```python
from build123d import *

# Parameters (mm, degrees)
F1_DEPTH = 25
F4_D     = 5.5
F3_R     = 11
F5_DEPTH = 4


with BuildPart() as f1:
    # F0 (on Front) → F1 (new body, symmetric)
    with BuildSketch(Plane.XZ):
        with BuildLine():
            Line((23.3431457505, 0), (0, 0))
            Line((0, 0), (0, -4))
            Line((0, -4), (25, -4))
            ThreePointArc((25, -4), (26.5307337295, -3.69551813), (27.8284271247, -2.8284271247))
            Line((27.8284271247, -2.8284271247), (148.0365799265, 117.379725677))
            Line((148.0365799265, 117.379725677), (145.2081528017, 120.2081528017))
            Line((145.2081528017, 120.2081528017), (26.1715728753, 1.1715728753))
            ThreePointArc((26.1715728753, 1.1715728753), (24.87387948, 0.30448187), (23.3431457505, 0))
        make_face()
    extrude(amount=F1_DEPTH, both=True)

    # F2: F1 across plane


with BuildPart() as f1_1:
    add(f1.part)
    add(f1.part.mirror(Plane.YZ))

    # F4 (through all)
    with Locations(Plane.XY):
        with Locations((-17.45, 0), (8.725, -15.112143296), (8.725, 15.112143296)):
            Hole(F4_D / 2)

    # F3 (on face) → F5 (cut, through all)
    with BuildSketch(Plane.XY):
        Circle(F3_R)
    extrude(amount=-F5_DEPTH, mode=Mode.SUBTRACT)


solid = f1_1.part
```
Build history of the part. All positions in model axes, mm. A direction names the side the tool comes from. Give positions to 0.01 mm unless a question says otherwise; leave off trailing zeros. Loops run counter-clockwise (first coordinate to the right, second up) from the corner with the lowest first, then second, coordinate; pieces in that order, holes last.
1) Probe line 1 along Y through (x, z) = (-17, -2); line 2 along X through (y, z) = (10.5, 93.5); line 3 along X through (y, z) = (-8.5, 24). List the from-to ranges inside material, lowest first.
Values follow:
line 1: y = -25 to -2.71, 2.71 to 25
line 2: x = -124.16 to -118.5, 118.5 to 124.16
line 3: x = -54.66 to -49, 49 to 54.66
2) 3-axis set-ups, long thin cutter, end or side, ignore diameter. For faces 4 (the face through (87, 0, 62)), 5 (the face through (11.5, -0.4, -4)): which of +Z, -Z, +X, -X, +Y, -Y reach the whole face in a straight line?
Values follow:
face 4: +Z, +Y, -Y
face 5: -Z, +X, -X, +Y, -Y
3) Band-saw the part on B-B on y = 0. List the corners of the cut face in (x, z).
Values follow:
outline: (-148.04, 117.38) - (-27.83, -2.83) arc R4 ccw to (-25, -4) - (-20.2, -4) - (-20.2, 0) - (-23.34, 0) arc R4 cw to (-26.17, 1.17) - (-145.21, 120.21) - close; (-14.7, -4) - (-11, -4) - (-11, 0) - (-14.7, 0) - close; (11, -4) - (25, -4) arc R4 ccw to (27.83, -2.83) - (148.04, 117.38) - (145.21, 120.21) - (26.17, 1.17) arc R4 cw to (23.34, 0) - (11, 0) - close
4) Drop flat-ended pins along their axis: P1, Ø5, axis at x = -64, y = -14, coming from the -Z side; P2, Ø1, axis at x = 89, y = -6, coming from the +Z side; P3, Ø3, axis at y = 9, z = 61.5, coming from the -X side; P4, Ø6.5, axis at x = -17.45, y = 0, coming from the -Z side. Give the stop position or say it passes through.
Values follow:
P1: stops at z = 30.84
P2: stops at z = 64.5
P3: stops at x = -93.66
P4: stops at z = -4
5) Band-saw the part on D-D on y = -22. List the corners of the cut face in (x, z), then the cut area to 3 significant figures.
Values follow:
outline: (-148.04, 117.38) - (-27.83, -2.83) arc R4 ccw to (-25, -4) - (25, -4) arc R4 ccw to (27.83, -2.83) - (148.04, 117.38) - (145.21, 120.21) - (26.17, 1.17) arc R4 cw to (23.34, 0) - (-23.34, 0) arc R4 cw to (-26.17, 1.17) - (-145.21, 120.21) - close
area: 1,570 mm2
6) Band-saw the part on C-C on z = 111. List the corners of the cut face in (x, y).
Values follow:
outline: (-141.66, -25) - (-136, -25) - (-136, 25) - (-141.66, 25) - close; (136, -25) - (141.66, -25) - (141.66, 25) - (136, 25) - close
7) Two-plate mould, pull along Y, no slides. Class faces 1 (the face through (9.083, -12.386, -2.028)), 2 (the face through (-87, 0, 62)), 3 (the face through (1, 25, -1)): released by +Y, released by -Y, zero draft, split by the parting line, or undercut.
Values follow:
face 1: undercut
face 2: zero draft
face 3: released by +Y
8) Band-saw the part on A-A on x = 0. List the corners of the cut face in (y, z).
Values follow:
outline: (-25, -4) - (-11, -4) - (-11, 0) - (-25, 0) - close; (11, -4) - (25, -4) - (25, 0) - (11, 0) - close
